from build123d import *

# Parameters (mm, degrees)
F1_DEPTH = 152.4
F2_R     = 5.08
F3_R     = 5.08


with BuildPart() as f1:
    # F0 (on Front) → F1 (new body)
    with BuildSketch(Plane.XZ):
        Polygon((76.2, 0), (0, 0), (-76.2, 0), (-76.2, -25.4), (0, -39.274979), (76.2, -25.4), align=None)
    extrude(amount=-F1_DEPTH)

    # F2
    f2_edges = [f1.edges().sort_by_distance(p)[0] for p in [
        (76.2, 76.2, 0),
        (0, 152.4, 0),
        (-76.2, 76.2, 0),
        (0, 0, 0),
    ]]
    fillet(f2_edges, radius=F2_R)

    # F3
    f3_edges = [f1.edges().sort_by_distance(p)[0] for p in [
        (76.2, 76.2, -25.4),
        (38.1, 0, -32.33749),
        (-38.1, 0, -32.33749),
        (38.1, 152.4, -32.33749),
        (-38.1, 152.4, -32.33749),
        (-76.2, 76.2, -25.4),
    ]]
    fillet(f3_edges, radius=F3_R)


solid = f1.part
Can you work these out from the model? Positions are in its coordinate system, mm. Round coordinates to 2 decimals unless told otherwise and drop trailing zeros. Order: outer loops, then holes, each group sorted by start corner. A loop starts at its lowest first (then second) coordinate and runs counter-clockwise, first axis right, second up. Notation, with made-up numbers: (77, 79.5) -> (82, 79.5) arc R16 cw to (82, 92.5) -> close; hole circle Ø1 at (33.5, -17). An arc over 180 degrees is marked (long way). Write each question's results on one line, items separated by ' | '. Start each with the question number.
Item 1: Please list where these lines run through material, in increasing order: L1, parallel to Y at x = 14, z = -32.5; L2, parallel to X at y = 25, z = -2; L3, parallel to Y at x = 11, z = -36.5.
Item 2: If we section it at A-A, the plane y = 31: Write out the boundary of the cut face in (x, z).
Item 3: Will these pins go through, and if not, where does the flat tip stop? pin 1 (8 mm diameter, centred on y = 102, z = -23.5, fed in from -X); pin 2 (4 mm diameter, centred on y = 87, z = -25, fed in from +X); pin 3 (5 mm diameter, centred on x = -39.5, z = -30.5, fed in from +Y).
Results:
1) L1: y = 0.08 to 152.32 | L2: x = -75.16 to 75.16 | L3: y = 2.41 to 149.99
2) outline: (-76.2, -21.16) arc R5.08 ccw to (-72.03, -26.16) -> (0, -39.27) -> (72.03, -26.16) arc R5.08 ccw to (76.2, -21.16) -> (76.2, -5.08) arc R5.08 ccw to (71.12, 0) -> (-71.12, 0) arc R5.08 ccw to (-76.2, -5.08) -> close
3) pin 1: stops at x = -76.2 | pin 2: stops at x = 75.86 | pin 3: stops at y = 152.3
